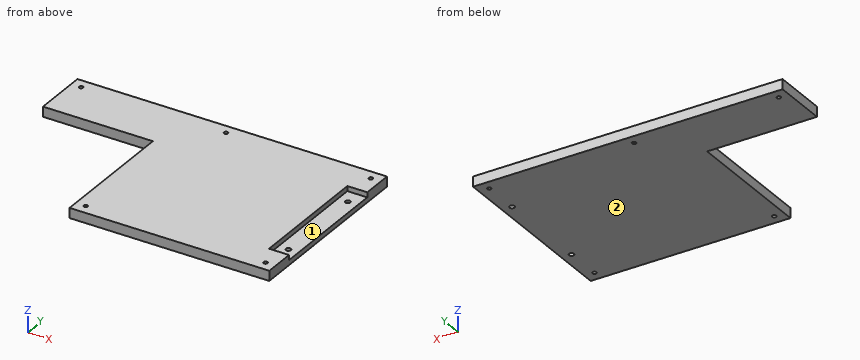
Autodesk Inventor part; units mm, degrees
ref_plane "YZ Plane" through (0, 0, 0) normal (1, 0, 0) x (0, 1, 0)
ref_plane "XZ Plane" through (0, 0, 0) normal (0, 1, 0) x (-1, 0, 0)
ref_plane "XY Plane" through (0, 0, 0) normal (0, 0, 1) x (1, 0, 0)
sketch "Sketch1" plane through (0, 0, 0) normal (0, 0, 1) x (1, 0, 0)
  line L0 (0, 0) -> (620, 0)
  line L1 (110, -188) -> (510, -188)
  line L2 (510, -188) -> (510, -55)
  line L3 (510, -55) -> (620, -55)
  line L4 (620, -55) -> (620, 0)
  line L5 (110, -188) -> (110, -55)
  line L6 (0, -55) -> (0, 0)
  line L7 (0, -55) -> (110, -55)
  point P0 (310, -188)
  point P1 (310, 0)
  dimension "d0" = 620
  dimension "d1" = 188
  dimension "d2" = 400
  dimension "d3" = 133
extrude "Extrusion1" add sketch "Sketch1" along normal blind 10
sketch "Sketch2" plane through (0, 0, 10) normal (0, 0, 1) x (1, 0, 0)
  line L0 (620, 0) -> (0, 0)
  line L1 (510, -188) -> (110, -188)
  line L2 (620, 0) -> (310, 0)
  line L3 (310, 0) -> (310, -188)
  line L4 (310, -188) -> (620, -188)
  line L5 (620, -188) -> (620, 0)
extrude "Extrusion2" cut sketch "Sketch2" against normal through all
sketch "Sketch3" plane through (0, 0, 10) normal (0, 0, 1) x (1, 0, 0)
  circle A0 centre (10, -10) radius 2
  line L0 (310, 0) -> (0, 0)
  line L1 (0, 0) -> (0, -55)
  circle A1 centre (155, -10) radius 2
  circle A2 centre (300, -10) radius 2
  line L2 (310, -188) -> (310, 0)
  line L3 (10, -10) -> (300, -10) construction
  circle A3 centre (120, -178) radius 2
  line L4 (110, -55) -> (110, -188)
  line L5 (110, -188) -> (310, -188)
  circle A4 centre (300, -178) radius 2
  dimension "d8" = 4
  dimension "d9" = 10
  dimension "d10" = 10
  dimension "d11" = 4
  dimension "d12" = 4
  dimension "d13" = 10
  dimension "d14" = 4
  dimension "d15" = 10
  dimension "d16" = 10
  dimension "d17" = 4
  dimension "d18" = 10
  dimension "d19" = 10
extrude "Extrusion3" cut sketch "Sketch3" against normal through all
sketch "Sketch6" plane through (0, 0, 10) normal (0, 0, 1) x (1, 0, 0)
  line L0 (310, -31.5) -> (290, -31.5)
  line L1 (290, -31.5) -> (290, -156.5)
  line L2 (290, -156.5) -> (310, -156.5)
  line L3 (310, -156.5) -> (310, -31.5)
  line L4 (310, -188) -> (310, 0)
  point P0 (0, 0)
  point P1 (310, -94)
  dimension "d42" = 20
  dimension "d43" = 125
extrude "Extrusion6" cut sketch "Sketch6" against normal blind 5
sketch "Sketch7" plane through (0, 0, 5) normal (0, 0, 1) x (1, 0, 0)
  line L0 (300, -46.5) -> (300, -141.5) construction
  circle A0 centre (300, -46.5) radius 2.5
  circle A1 centre (300, -141.5) radius 2.5
  line L1 (310, -31.5) -> (310, -156.5)
  point P0 (0, 0)
  point P1 (300, -94)
  point P2 (310, -94)
  dimension "d46" = 5
  dimension "d47" = 5
  dimension "d48" = 10
  dimension "d49" = 95
extrude "Extrusion7" cut sketch "Sketch7" against normal through all
properties part number "SP001b" material "ABS Plastic"
Check sheet for the modelled part. Datum: model origin and axes. Units: mm. Face numbers are marked on the shaded views. A direction names the side the tool comes from. Give positions to 0.01 mm unless a question says otherwise; leave off trailing zeros. Write each loop counter-clockwise with the first axis right and the second up, starting at its lowest first coordinate (ties: lowest second). Pieces come first, ordered by that corner, then holes. Notation, with made-up numbers: (83, 60) - (118, 60) arc R28 ccw to (118, 81) - close; hole circle Ø3 at (34, 24). An arc over 180 degrees is marked (long way). Answer as a JSON object with one key per item and string values. Group by question number.
1) Sectioned sample at A-A (z = 2). Record the cut outline in (x, y), then the cut area to 3 significant figures.
2) Depth check by flat-ended pin: P1, Ø2.5, axis at x = 300, y = -178, coming from the -Z side; P2, Ø8, axis at x = 300, y = -141.5, coming from the +Z side; P3, Ø3, axis at x = 78.5, z = 5.5, coming from the -Y side. Enter the tip coordinate at first touch or a pass-through.
3) Thickness scan on probe 1 along Y at (x, z) = (300, 2.4); probe 2 along X at (y, z) = (-178, 4.25); probe 3 along X at (y, z) = (-141.5, 1.05). Record the ranges inside material, lowest first. Write a range as from..to.
4) Sectioned sample at B-B (y = -123). Record the cut outline in (x, z).
5) Sectioned sample at C-C (x = 82.5). Record the cut outline in (y, z), then the cut area to 3 significant figures.
6) Access from +Z, -Z, +X, -X, +Y, -Y to the whole of each face (thin tool, end or side, straight path). Record for the marked faces 1 and 2.
Geometry results:
{
 "1": {"outline": "(0, -55) - (110, -55) - (110, -188) - (310, -188) - (310, 0) - (0, 0) - close; hole circle Ø4 at (10, -10); hole circle Ø4 at (120, -178); hole circle Ø4 at (155, -10); hole circle Ø5 at (300, -141.5); hole circle Ø5 at (300, -46.5); hole circle Ø4 at (300, -178); hole circle Ø4 at (300, -10)", "area": "43,500 mm^2"},
 "2": {"P1": "passes through", "P2": "stops at z = 5", "P3": "stops at y = -55"},
 "3": {"probe 1": "y = -188..-180, -176..-144, -139..-49, -44..-12, -8..0", "probe 2": "x = 110..118, 122..298, 302..310", "probe 3": "x = 110..297.5, 302.5..310"},
 "4": {"outline": "(110, 0) - (310, 0) - (310, 5) - (290, 5) - (290, 10) - (110, 10) - close"},
 "5": {"outline": "(-55, 0) - (0, 0) - (0, 10) - (-55, 10) - close", "area": "550 mm^2"},
 "6": {"face 1": "+Z, +X", "face 2": "-Z, +X, -X, +Y, -Y"}
}
